For this review, take the finished solid that the model builds, in its own axes (mm). A direction names the side the tool comes from. Coordinates: 2 decimals unless noted, no trailing zeros. Order: outer loops, then holes, each group sorted by start corner. A loop starts at its lowest first (then second) coordinate and runs counter-clockwise, first axis right, second up. Notation, with made-up numbers: (29, -30.5) - (56, -30.5) arc R24 cw to (56, 4.5) - close; hole circle Ø8 at (51.25, 73.25). An arc over 180 degrees is marked (long way). One line per item, written item: value. Start each with the question number.
(1) For faces 4 (the flat face through (-10, 0, 0)), 5 (the flat face through (15.199, 2, -7)), 6 (the flat face through (5.799, 2, 0)), 7 (the flat face through (-14, 2, 7.869)), 8 (the flat face through (-17.972, 2, 4)), list the 3-axis set-ups (+Z, -Z, +X, -X, +Y, -Y) from which the entire face can be reached by the end or side of a thin tool; tool diameter is ignored.
(2) Consider section A-A on z = 0. Write out the cut boundary in (x, y), then the cut area to 3 significant figures.
(3) Consider section C-C on y = -5.5. Write out the cut boundary in (x, z), then the cut area to 3 significant figures.
(4) Consider section D-D on z = -10.5. Write out the cut boundary in (x, y), then the cut area to 3 significant figures.
(5) To check wall thickness, follow line 1 along X through (y, z) = (1.5, -7.5); line 2 along Y through (x, z) = (-15.5, 0); line 3 along Y through (x, z) = (13, 1). State the ranges of each line that lie inside material, in increasing order.
(6) Clearance check with flat-ended pins moving along their axes: pin 1 (0.5 mm diameter, centred on x = -1.5, y = 2, fed in from +Z); pin 2 (10 mm diameter, centred on y = -6, z = -2, fed in from +X); pin 3 (1.5 mm diameter, centred on x = -1, z = 4.5, fed in from -Y); pin 4 (0.6 mm diameter, centred on y = 2, z = -4.5, fed in from -X). State where each tip first meets the part, or that it passes through.
(7) Mouldability with a two-part tool opening along X and no side actions: class faces 1 (the flat face through (10, 0, 0)), 2 (the flat face through (-1.6, 2.5, 3.141)), 3 (the flat face through (-13.81, 2.46, 9.4)) as released by +X, released by -X, zero draft, split by the parting line, or undercut.
(8) Consider section B-B on x = 0.5. Write out the cut boundary in (y, z).
```python
from build123d import *

# Parameters (mm, degrees)
CROQUIS2_R                = 1.779687177
SALIENTE_EXTRUIR1_DEPTH   = 5
SALIENTE_EXTRUIR1_2_DEPTH = 5
SALIENTE_EXTRUIR1_3_DEPTH = 5
SALIENTE_EXTRUIR1_4_DEPTH = 5
SALIENTE_EXTRUIR1_5_DEPTH = 5
SALIENTE_EXTRUIR1_6_DEPTH = 5
SALIENTE_EXTRUIR1_7_DEPTH = 5
SALIENTE_EXTRUIR1_8_DEPTH = 5
SALIENTE_EXTRUIR1_9_DEPTH = 5
CROQUIS3_W                = 40.052022685
CROQUIS3_H                = 20
SALIENTE_EXTRUIR2_DEPTH   = 3
REDONDEO1_R               = 2
CROQUIS4_W                = 40.052022685
CROQUIS4_H                = 25
SALIENTE_EXTRUIR3_DEPTH   = 3
CHAFL_N1_SIZE             = 1


with BuildPart() as part:
    # Croquis2 → Saliente-Extruir1 (new body)
    with BuildSketch(Plane(origin=(0, 0, 0), x_dir=(1, 0, 0), z_dir=(0, 1, 0))):
        with Locations(Location((-10.039017014, 0, 0), (0, 0, 90))):
            Circle(CROQUIS2_R)
    extrude(amount=SALIENTE_EXTRUIR1_DEPTH)



with BuildPart() as body_2:
    # Croquis2 → Saliente-Extruir1 2 (new body)
    with BuildSketch(Plane(origin=(0, 0, 0), x_dir=(1, 0, 0), z_dir=(0, 1, 0))):
        with Locations(Location((9.986994329, 0, 0), (0, 0, 270))):
            Circle(CROQUIS2_R)
    extrude(amount=SALIENTE_EXTRUIR1_2_DEPTH)


with BuildPart() as body_3:
    # Croquis2 → Saliente-Extruir1 3 (new body)
    with BuildSketch(Plane(origin=(0, 0, 0), x_dir=(1, 0, 0), z_dir=(0, 1, 0))):
        Polygon((5.614984779, 10), (14.359003879, 10), (13.134466077, 8.775462198), (13.134466077, 7.868577354), (15.198808852, 7.868577354), (15.198808852, 6.711119422), (12.681851378, 4.194161948), (7.292137279, 4.194161948), (4.775179805, 6.711119422), (4.775179805, 7.868577354), (6.839522581, 7.868577354), (6.839522581, 8.775462198), align=None)
    extrude(amount=SALIENTE_EXTRUIR1_3_DEPTH)


with BuildPart() as body_4:
    # Croquis2 → Saliente-Extruir1 4 (new body)
    with BuildSketch(Plane(origin=(0, 0, 0), x_dir=(1, 0, 0), z_dir=(0, 1, 0))):
        Polygon((20, 4.155027818), (20, -4.155027818), (18.985761672, -3.14078949), (17.919495795, -3.14078949), (17.919495795, -5.172992947), (16.531532714, -5.172992947), (14.175115642, -2.816575874), (14.175115642, 2.816575874), (16.531532714, 5.172992947), (17.919495795, 5.172992947), (17.919495795, 3.14078949), (18.985761672, 3.14078949), align=None)
    extrude(amount=SALIENTE_EXTRUIR1_4_DEPTH)


with BuildPart() as body_5:
    # Croquis2 → Saliente-Extruir1 5 (new body)
    with BuildSketch(Plane(origin=(0, 0, 0), x_dir=(1, 0, 0), z_dir=(0, 1, 0))):
        Polygon((-0.026011343, 4.155027818), (-1.040249671, 3.14078949), (-2.106515548, 3.14078949), (-2.106515548, 5.172992947), (-3.494478629, 5.172992947), (-5.850895701, 2.816575874), (-5.850895701, -2.816575874), (-3.494478629, -5.172992947), (-2.106515548, -5.172992947), (-2.106515548, -3.14078949), (-1.040249671, -3.14078949), (-0.026011343, -4.155027818), (0.988226986, -3.14078949), (2.054492862, -3.14078949), (2.054492862, -5.172992947), (3.442455943, -5.172992947), (5.798873016, -2.816575874), (5.798873016, 2.816575874), (3.442455943, 5.172992947), (2.054492862, 5.172992947), (2.054492862, 3.14078949), (0.988226986, 3.14078949), align=None)
    extrude(amount=SALIENTE_EXTRUIR1_5_DEPTH)


with BuildPart() as body_6:
    # Croquis2 → Saliente-Extruir1 6 (new body)
    with BuildSketch(Plane(origin=(0, 0, 0), x_dir=(1, 0, 0), z_dir=(0, 1, 0))):
        Polygon((4.775179805, -6.711119422), (7.292137279, -4.194161948), (12.681851378, -4.194161948), (15.198808852, -6.711119422), (15.198808852, -7.868577354), (13.134466077, -7.868577354), (13.134466077, -8.775462198), (14.359003879, -10), (5.614984779, -10), (6.839522581, -8.775462198), (6.839522581, -7.868577354), (4.775179805, -7.868577354), align=None)
    extrude(amount=SALIENTE_EXTRUIR1_6_DEPTH)


with BuildPart() as body_7:
    # Croquis2 → Saliente-Extruir1 7 (new body)
    with BuildSketch(Plane(origin=(0, 0, 0), x_dir=(1, 0, 0), z_dir=(0, 1, 0))):
        Polygon((-12.733874064, -4.194161948), (-7.344159964, -4.194161948), (-4.82720249, -6.711119422), (-4.82720249, -7.868577354), (-6.891545266, -7.868577354), (-6.891545266, -8.775462198), (-5.667007464, -10), (-14.411026564, -10), (-13.186488762, -8.775462198), (-13.186488762, -7.868577354), (-15.250831538, -7.868577354), (-15.250831538, -6.711119422), align=None)
    extrude(amount=SALIENTE_EXTRUIR1_7_DEPTH)


with BuildPart() as body_8:
    # Croquis2 → Saliente-Extruir1 8 (new body)
    with BuildSketch(Plane(origin=(0, 0, 0), x_dir=(1, 0, 0), z_dir=(0, 1, 0))):
        Polygon((-16.583555399, -5.172992947), (-14.227138327, -2.816575874), (-14.227138327, 2.816575874), (-16.583555399, 5.172992947), (-17.97151848, 5.172992947), (-17.97151848, 3.14078949), (-19.037784357, 3.14078949), (-20.052022685, 4.155027818), (-20.052022685, -4.155027818), (-19.037784357, -3.14078949), (-17.97151848, -3.14078949), (-17.97151848, -5.172992947), align=None)
    extrude(amount=SALIENTE_EXTRUIR1_8_DEPTH)


with BuildPart() as body_9:
    # Croquis2 → Saliente-Extruir1 9 (new body)
    with BuildSketch(Plane(origin=(0, 0, 0), x_dir=(1, 0, 0), z_dir=(0, 1, 0))):
        Polygon((-5.667007464, 10), (-6.891545266, 8.775462198), (-6.891545266, 7.868577354), (-4.82720249, 7.868577354), (-4.82720249, 6.711119422), (-7.344159964, 4.194161948), (-12.733874064, 4.194161948), (-15.250831538, 6.711119422), (-15.250831538, 7.868577354), (-13.186488762, 7.868577354), (-13.186488762, 8.775462198), (-14.411026564, 10), align=None)
    extrude(amount=SALIENTE_EXTRUIR1_9_DEPTH)


with BuildPart() as part_1:
    add(part.part)

    add(body_2.part)  # Saliente-Extruir2 merges body 2

    add(body_3.part)  # Saliente-Extruir2 merges body 3

    add(body_4.part)  # Saliente-Extruir2 merges body 4

    add(body_5.part)  # Saliente-Extruir2 merges body 5

    add(body_6.part)  # Saliente-Extruir2 merges body 6

    add(body_7.part)  # Saliente-Extruir2 merges body 7

    add(body_8.part)  # Saliente-Extruir2 merges body 8

    add(body_9.part)  # Saliente-Extruir2 merges body 9
    # Croquis3 → Saliente-Extruir2 (add)
    with BuildSketch(Plane(origin=(0, 5, 0), x_dir=(1, 0, 0), z_dir=(0, 1, 0))):
        with Locations((-0.026011343, 0)):
            Rectangle(CROQUIS3_W, CROQUIS3_H)
    extrude(amount=SALIENTE_EXTRUIR2_DEPTH)

    # Redondeo1
    redondeo1_edges = [part_1.edges().sort_by_distance(p)[0] for p in [
        (-20.052022685, 8, 0),
        (-0.026011343, 8, 10),
        (20, 8, 0),
        (-0.026011343, 8, -10),
    ]]
    fillet(redondeo1_edges, radius=REDONDEO1_R)

    # Croquis4 → Saliente-Extruir3 (add)
    with BuildSketch(Plane(origin=(0, 0, -10), x_dir=(-1, 0, 0), z_dir=(0, 0, -1))):
        with Locations((0.026011343, -6.5)):
            Rectangle(CROQUIS4_W, CROQUIS4_H)
    extrude(amount=SALIENTE_EXTRUIR3_DEPTH)

    # Chaflán1
    chafl_n1_edges = [part_1.edges().sort_by_distance(p)[0] for p in [
        (20, -6.5, -13),
        (-0.026011343, -19, -13),
        (-20.052022685, -6.5, -13),
        (-0.026011343, 6, -13),
    ]]
    chamfer(chafl_n1_edges, length=CHAFL_N1_SIZE)


solid = part_1.part
```
Geometry check:
1. face 4: +Z, +X, -X, -Y
1. face 5: +X, -Y
1. face 6: -Y
1. face 7: -X, -Y
1. face 8: +Z, -Y
2. outline: (-20.05, 0) - (-14.23, 0) - (-14.23, 5) - (-11.82, 5) - (-11.82, 0) - (-8.26, 0) - (-8.26, 5) - (-5.85, 5) - (-5.85, 0) - (5.8, 0) - (5.8, 5) - (8.21, 5) - (8.21, 0) - (11.77, 0) - (11.77, 5) - (14.18, 5) - (14.18, 0) - (20, 0) - (20, 6) arc R2 ccw to (18, 8) - (-18.05, 8) arc R2 ccw to (-20.05, 6) - close
2. area: 271 mm^2
3. outline: (-20.05, -12) - (-19.05, -13) - (19, -13) - (20, -12) - (20, -10) - (-20.05, -10) - close
3. area: 119 mm^2
4. outline: (-20.05, -19) - (20, -19) - (20, 6) - (-20.05, 6) - close
4. area: 1,000 mm^2
5. line 1: x = -15.25 to -4.83, 4.78 to 15.2
5. line 2: y = 0 to 8
5. line 3: y = 5 to 8
6. pin 1: stops at z = 3.14
6. pin 2: passes through
6. pin 3: stops at y = 5
6. pin 4: stops at x = -17.97
7. face 1: zero draft
7. face 2: undercut
7. face 3: released by -X
8. outline: (-19, -12) - (-18, -13) - (5, -13) - (6, -12) - (6, -10) arc R2 ccw to (8, -8) - (8, 8) arc R2 ccw to (6, 10) - (5, 10) - (5, 3.63) - (0, 3.63) - (0, -3.63) - (5, -3.63) - (5, -10) - (-19, -10) - close
